Verification items for this drawing (mm, ordinates from the low corner). A direction names the side the tool comes from. Round coordinates to 2 decimals unless told otherwise and drop trailing zeros. Write each loop counter-clockwise with the first axis right and the second up, starting at its lowest first coordinate (ties: lowest second). Pieces come first, ordered by that corner, then holes. Notation, with made-up numbers: M 29.5,20 L 61.5,20 A24 cw 61.5,52 Z; hole C 44,36.5 d6. An arc over 180 degrees is marked long. Write each question's results on one line, items separated by ' | '.
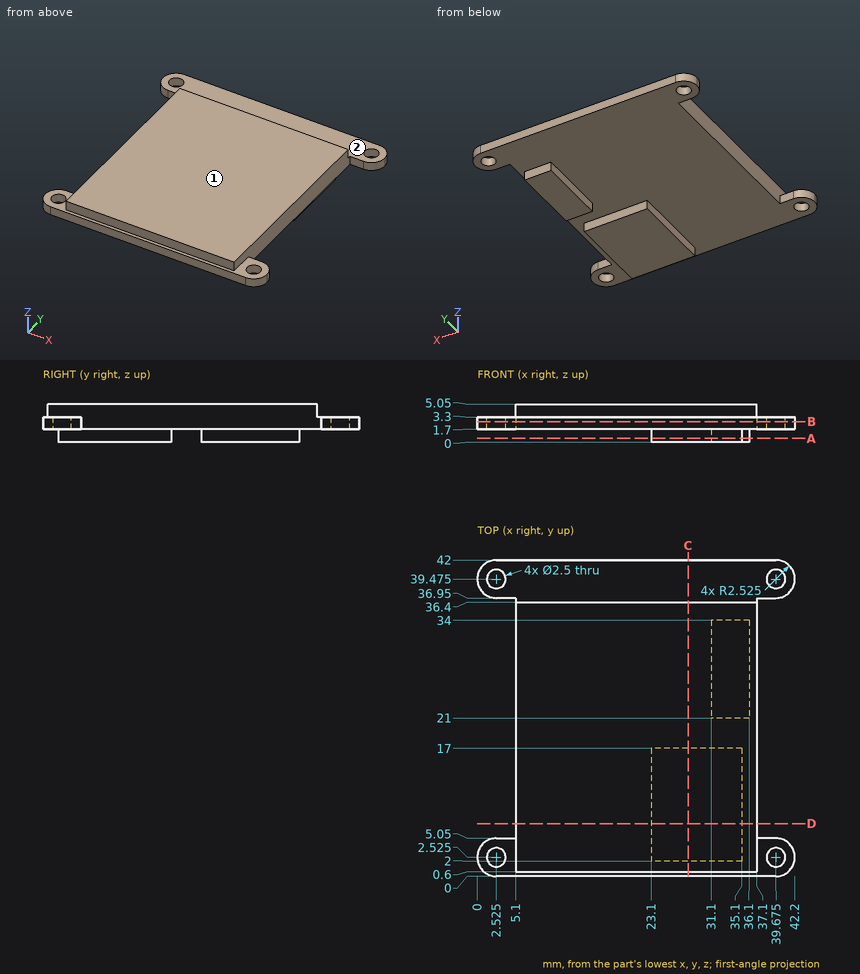
1) Material ranges on line 1 (Y direction, x = 2.5, z = 3); line 2 (Y direction, x = 4.5, z = 2); line 3 (Z direction, x = 20, y = 40), recorded low to high. Write a range as [from, to].
Calculated:
line 1: y = [0, 1.28], [3.77, 5.05], [36.95, 38.23], [40.72, 42] | line 2: y = [0, 5.05], [36.95, 42] | line 3: z = [1.7, 3.3]
2) Depth check by flat-ended pin: P1, Ø0.9, axis at y = 12.5, z = 1, coming from the -X side; P2, Ø1.5, axis at x = 8, y = 17, coming from the -Z side; P3, Ø0.5, axis at x = 34.5, z = 1, coming from the +Y side; P4, Ø2, axis at x = 39.675, y = 2.525, coming from the +Z side. Enter the tip coordinate at first touch or a pass-through.
Calculated:
P1: stops at x = 23.1 | P2: stops at z = 1.7 | P3: stops at y = 34 | P4: passes through
3) Sectioned sample at C-C, the plane x = 28. Record the cut outline in (y, z), and give its area (3 significant figures).
Calculated:
outline: M 0,1.7 L 2,1.7 L 2,0 L 17,0 L 17,1.7 L 42,1.7 L 42,3.3 L 36.4,3.3 L 36.4,5.05 L 0.6,5.05 L 0.6,3.3 L 0,3.3 Z | area: 155 mm²
4) Sectioned sample at A-A, the plane z = 0.5. Record the cut outline in (x, y).
Calculated:
outline: M 23.1,2 L 35.1,2 L 35.1,17 L 23.1,17 Z; M 31.1,21 L 36.1,21 L 36.1,34 L 31.1,34 Z
5) Access from +Z, -Z, +X, -X, +Y, -Y to the whole of each face (thin tool, end or side, straight path). Record for the marked faces 1 and 2.
Calculated:
face 1: +Z, +X, -X, +Y, -Y | face 2: +Z, +X, -X, +Y
6) Sectioned sample at D-D, the plane y = 7. Record the cut outline in (x, z).
Calculated:
outline: M 5.1,1.7 L 23.1,1.7 L 23.1,0 L 35.1,0 L 35.1,1.7 L 37.1,1.7 L 37.1,5.05 L 5.1,5.05 Z
7) Sectioned sample at B-B, the plane z = 2.7. Record the cut outline in (x, y) (3 decimals).
Calculated:
outline: M 0,2.525 A2.525 ccw 2.525,0 L 39.675,0 A2.525 ccw 42.2,2.525 A2.525 ccw 39.675,5.05 L 37.1,5.05 L 37.1,36.95 L 39.675,36.95 A2.525 ccw 42.2,39.475 A2.525 ccw 39.675,42 L 2.525,42 A2.525 ccw 0,39.475 A2.525 ccw 2.525,36.95 L 5.1,36.95 L 5.1,5.05 L 2.525,5.05 A2.525 ccw Z; hole C 2.525,2.525 d2.5; hole C 2.525,39.475 d2.5; hole C 39.675,2.525 d2.5; hole C 39.675,39.475 d2.5
